The model under review builds one solid part; all positions refer to its coordinate system, in mm. Face numbers are marked on the shaded views. A direction names the side the tool comes from. Round coordinates to 2 decimals unless told otherwise and drop trailing zeros. Loops run counter-clockwise (first coordinate to the right, second up) from the corner with the lowest first, then second, coordinate; pieces in that order, holes last. Notation, with made-up numbers: M 43.25,-17 L 102.25,-17 A15 cw 102.25,3 Z; hole C -28.5,-23 d3. An arc over 180 degrees is marked long. Answer as a JSON object with one key per item and string values. Group by question number.
Item 1: Consider section C-C (y = -37.5). Give the boundary of the cut face in (x, z).
Item 2: To check wall thickness, follow line 1 (X direction, y = -32, z = 1.25); line 2 (Y direction, x = 28, z = 1); line 3 (X direction, y = -30, z = 5.5). State the ranges of each line that lie inside material, in increasing order.
Item 3: Tool access review of the marked faces 1, 2, 3, 4 and 5: name each direction out of +Z, -Z, +X, -X, +Y, -Y from which nothing blocks a thin tool from reaching the whole face with its end or side.
Item 4: The part is to be moulded in two halves that separate along Y. For the marked faces 6, 7 and 8, say which applies: +Y half, -Y half, draft (parallel to the pull), parting line (faces both ways), or undercut.
Item 5: Consider section D-D (z = 4.5). State how many separate pieces and enclosed holes the cut face has, and give its area (3 significant figures).
Item 6: Consider section B-B (x = -23.5). Give the boundary of the cut face in (y, z).
Item 7: Consider section A-A (y = -12.5). Give the boundary of the cut face in (x, z), and give its area (3 significant figures).
Item 8: Insertion check: P1, Ø3, axis at x = -49, z = 2.5, coming from the -Y side; P2, Ø3, axis at y = -14, z = 2.5, coming from the -X side; P3, Ø6, axis at x = 27.5, y = 6.5, coming from the +Z side; P4, Ø3, axis at x = -21.5, z = 2, coming from the -Y side. Each pin has a flat end and moves straight along its axis. Give the tip position at first contact, or say it passes through.
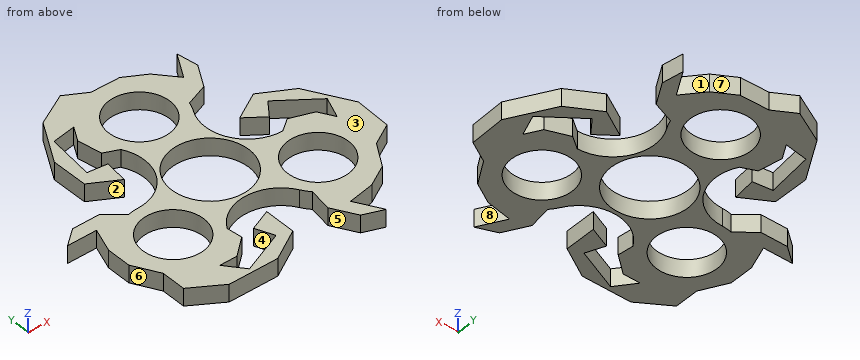
```python
from build123d import *

# Parameters (mm, degrees)
F0_R     = 11.049
F0_R_2   = 13.97
F1_DEPTH = 6.35


with BuildPart() as f1:
    # F0 (on Top) → F1 (new body)
    with BuildSketch(Plane.XY):
        with BuildLine():
            ThreePointArc((26.396454, 0), (13.198227, 7.62), (13.198227, 22.86))
            ThreePointArc((13.198227, 22.86), (14.009272, 24.480176), (14.622308, 26.185155))
            Line((14.622308, 26.185155), (22.382144, 29.153406))
            Line((22.382144, 29.153406), (27.188946, 37.479031))
            Line((27.188946, 37.479031), (25.972238, 44.985235))
            Line((25.972238, 44.985235), (20.700261, 35.853904))
            Line((20.700261, 35.853904), (14.596639, 42.95875))
            Line((14.596639, 42.95875), (7.07672, 47.300377))
            Line((7.07672, 47.300377), (-3.192702, 47.499965))
            Line((-3.192702, 47.499965), (-10.71262, 51.841591))
            Line((-10.71262, 51.841591), (-22.048165, 45.852972))
            Line((-22.048165, 45.852972), (-30.886479, 30.544563))
            Line((-30.886479, 30.544563), (-30.751104, 17.754158))
            Line((-30.751104, 17.754158), (-21.025084, 12.138838))
            Line((-21.025084, 12.138838), (-20.050264, 20.312221))
            Line((-20.050264, 20.312221), (-27.004857, 21.141678))
            Line((-27.004857, 21.141678), (-25.046949, 37.557762))
            Line((-25.046949, 37.557762), (-16.771019, 38.867205))
            Line((-16.771019, 38.867205), (-19.872182, 33.495833))
            Line((-19.872182, 33.495833), (-18.294169, 25.064847))
            Line((-18.294169, 25.064847), (-13.198227, 22.86))
            ThreePointArc((-13.198227, 22.86), (-13.198227, 7.62), (-26.396454, 0))
            ThreePointArc((-26.396454, 0), (-28.205091, -0.107702), (-29.988163, -0.429287))
            Line((-29.988163, -0.429287), (-36.438663, 4.806802))
            Line((-36.438663, 4.806802), (-46.052266, 4.806802))
            Line((-46.052266, 4.806802), (-51.944476, 0))
            Line((-51.944476, 0), (-41.400522, 0))
            Line((-41.400522, 0), (-44.501688, -8.838315))
            Line((-44.501688, -8.838315), (-44.501688, -17.52157))
            Line((-44.501688, -17.52157), (-39.539825, -26.514944))
            Line((-39.539825, -26.514944), (-39.539825, -35.198197))
            Line((-39.539825, -35.198197), (-28.685756, -42.020757))
            Line((-28.685756, -42.020757), (-11.009128, -42.020757))
            Line((-11.009128, -42.020757), (0, -35.508316))
            Line((0, -35.508316), (0, -24.277676))
            Line((0, -24.277676), (-7.565767, -27.520148))
            Line((-7.565767, -27.520148), (-4.806802, -33.957731))
            Line((-4.806802, -33.957731), (-20.002501, -40.470175))
            Line((-20.002501, -40.470175), (-25.274477, -33.957731))
            Line((-25.274477, -33.957731), (-19.072151, -33.957731))
            Line((-19.072151, -33.957731), (-12.559709, -28.375639))
            Line((-12.559709, -28.375639), (-13.198227, -22.86))
            ThreePointArc((-13.198227, -22.86), (0, -15.24), (13.198227, -22.86))
            ThreePointArc((13.198227, -22.86), (14.195818, -24.372474), (15.365855, -25.755868))
            Line((15.365855, -25.755868), (14.056519, -33.960209))
            Line((14.056519, -33.960209), (18.86332, -42.285833))
            Line((18.86332, -42.285833), (25.972238, -44.985235))
            Line((25.972238, -44.985235), (20.700261, -35.853904))
            Line((20.700261, -35.853904), (29.905049, -34.120435))
            Line((29.905049, -34.120435), (37.424968, -29.778808))
            Line((37.424968, -29.778808), (42.732527, -20.985021))
            Line((42.732527, -20.985021), (50.252445, -16.643395))
            Line((50.252445, -16.643395), (50.733921, -3.832215))
            Line((50.733921, -3.832215), (41.895607, 11.476194))
            Line((41.895607, 11.476194), (30.751104, 17.754158))
            Line((30.751104, 17.754158), (21.025084, 12.138838))
            Line((21.025084, 12.138838), (27.616031, 7.207928))
            Line((27.616031, 7.207928), (31.811659, 12.816053))
            Line((31.811659, 12.816053), (45.049451, 2.912414))
            Line((45.049451, 2.912414), (42.045496, -4.909474))
            Line((42.045496, -4.909474), (38.944333, 0.461898))
            Line((38.944333, 0.461898), (30.853878, 3.310792))
            Line((30.853878, 3.310792), (26.396454, 0))
        make_face()
        with Locations((-26.396454, -15.24)):
            Circle(F0_R, mode=Mode.SUBTRACT)
        Circle(F0_R_2, mode=Mode.SUBTRACT)
        with Locations((26.396454, -15.24)):
            Circle(F0_R, mode=Mode.SUBTRACT)
        with Locations((0, 30.48)):
            Circle(F0_R, mode=Mode.SUBTRACT)
    extrude(amount=F1_DEPTH)


solid = f1.part
```
Geometry results:
{
 "1": {"outline": "M -35.88,0 L -22.41,0 L -22.41,6.35 L -35.88,6.35 Z; M -13.07,0 L -3.37,0 L -3.37,6.35 L -13.07,6.35 Z; M 16.1,0 L 21.65,0 L 21.65,6.35 L 16.1,6.35 Z"},
 "2": {"line 1": "x = -39.54 to -16.79, -5.65 to 0, 14.37 to 33.58", "line 2": "y = -34.48 to -26.17, -4.31 to 1.19, 7.72 to 16.17", "line 3": "x = -39.54 to -14.45, -6.5 to 0, 14.69 to 37.04"},
 "3": {"face 1": "+Z, -Z, +Y", "face 2": "+Z, -Z, -X", "face 3": "+Z, +X, -X, +Y, -Y", "face 4": "+Z, -Z", "face 5": "+Z, -Z, -Y"},
 "4": {"face 6": "-Y half", "face 7": "+Y half", "face 8": "undercut"},
 "5": {"separate pieces": "1", "enclosed holes": "4", "area": "3,010 mm^2"},
 "6": {"outline": "M -42.02,0 L -36.15,0 L -36.15,6.35 L -42.02,6.35 Z; M -33.96,0 L -25.9,0 L -25.9,6.35 L -33.96,6.35 Z; M -4.58,0 L 0.28,0 L 0.28,6.35 L -4.58,6.35 Z; M 13.57,0 L 20.72,0 L 20.72,6.35 L 13.57,6.35 Z; M 37.8,0 L 43.34,0 L 43.34,6.35 L 37.8,6.35 Z"},
 "7": {"outline": "M -44.5,0 L -37.1,0 L -37.1,6.35 L -44.5,6.35 Z; M -15.69,0 L -6.24,0 L -6.24,6.35 L -15.69,6.35 Z; M 6.24,0 L 15.69,0 L 15.69,6.35 L 6.24,6.35 Z; M 37.1,0 L 50.41,0 L 50.41,6.35 L 37.1,6.35 Z", "area": "252 mm^2"},
 "8": {"P1": "stops at y = 0", "P2": "stops at x = -44.5", "P3": "stops at z = 6.35", "P4": "stops at y = -42.02"}
}
